```python
from build123d import *

# Parameters (mm, degrees)
SKETCH1_W           = 45
SKETCH1_H           = 45
SKETCH1_R           = 9
SKETCH1_R_2         = 2
BOSS_EXTRUDE1_DEPTH = 15
SKETCH2_R           = 1.65
CUT_EXTRUDE1_DEPTH  = 15
SKETCH3_R           = 3
CUT_EXTRUDE2_DEPTH  = 8
CHAMFER1_SIZE       = 2
SKETCH4_R           = 11.2
CUT_EXTRUDE3_DEPTH  = 2
ECHELLE1_SCALE      = 2
ECHELLE2_SCALE      = 0.25


with BuildPart() as part:
    # Sketch1 → Boss-Extrude1 (new body)
    with BuildSketch(Plane.XY):
        Rectangle(SKETCH1_W, SKETCH1_H)
        Circle(SKETCH1_R, mode=Mode.SUBTRACT)
        with Locations((-17.5, 17.5)):
            Circle(SKETCH1_R_2, mode=Mode.SUBTRACT)
        with Locations((17.5, 17.5)):
            Circle(SKETCH1_R_2, mode=Mode.SUBTRACT)
        with Locations((17.5, -17.5)):
            Circle(SKETCH1_R_2, mode=Mode.SUBTRACT)
        with Locations((-17.5, -17.5)):
            Circle(SKETCH1_R_2, mode=Mode.SUBTRACT)
    extrude(amount=BOSS_EXTRUDE1_DEPTH)

    # Sketch2 → Cut-Extrude1 (cut)
    with BuildSketch(Plane.XY.offset(15)):
        with Locations((9.899494937, 9.899494937)):
            Circle(SKETCH2_R)
        with Locations((9.899494937, -9.899494937)):
            Circle(SKETCH2_R)
        with Locations((-9.899494937, -9.899494937)):
            Circle(SKETCH2_R)
        with Locations((-9.899494937, 9.899494937)):
            Circle(SKETCH2_R)
    extrude(amount=-CUT_EXTRUDE1_DEPTH, mode=Mode.SUBTRACT)

    # Sketch3 → Cut-Extrude2 (cut)
    with BuildSketch(Plane.XY.offset(15)):
        with Locations((9.899494937, 9.899494937)):
            Circle(SKETCH3_R)
        with Locations((9.899494937, -9.899494937)):
            Circle(SKETCH3_R)
        with Locations((-9.899494937, -9.899494937)):
            Circle(SKETCH3_R)
        with Locations((-9.899494937, 9.899494937)):
            Circle(SKETCH3_R)
    extrude(amount=-CUT_EXTRUDE2_DEPTH, mode=Mode.SUBTRACT)

    # Chamfer1
    chamfer1_edges = [part.edges().sort_by_distance(p)[0] for p in [
        (22.5, -22.5, 7.5),
        (-22.5, -22.5, 7.5),
        (-22.5, 22.5, 7.5),
        (22.5, 22.5, 7.5),
    ]]
    chamfer(chamfer1_edges, length=CHAMFER1_SIZE)

    # Sketch4 → Cut-Extrude3 (cut)
    with BuildSketch(Plane(origin=(0, 0, 0), x_dir=(-1, 0, 0), z_dir=(0, 0, -1))):
        Circle(SKETCH4_R)
    extrude(amount=-CUT_EXTRUDE3_DEPTH, mode=Mode.SUBTRACT)


with BuildPart() as part_1:
    # Echelle1: scaled about (0, 0, 7.483766611)
    add(part.part.scale(ECHELLE1_SCALE).moved(Location((0, 0, -7.483766611))))


with BuildPart() as part_2:
    # Echelle2: scaled about (0, 0, 7.483766612)
    add(part_1.part.scale(ECHELLE2_SCALE).moved(Location((0, 0, 5.612824959))))


solid = part_2.part
```
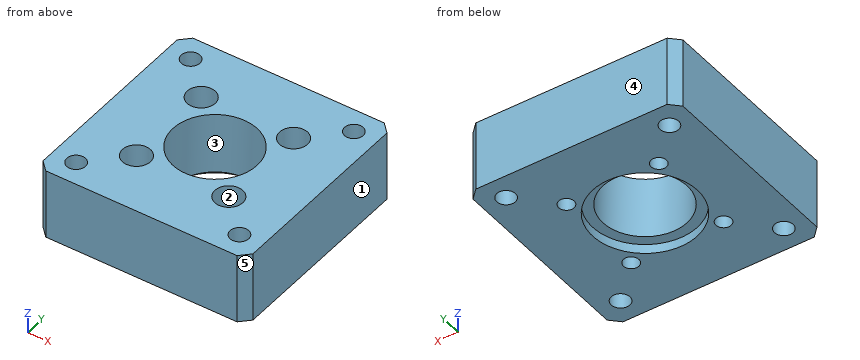
Input: part model. Units: mm. Frame: model coordinates. Face numbers are marked on the shaded views. A direction names the side the tool comes from. Coordinates: 2 decimals unless noted, no trailing zeros. Write each loop counter-clockwise with the first axis right and the second up, starting at its lowest first coordinate (ties: lowest second). Pieces come first, ordered by that corner, then holes.
1) Section C-C on x = 8.75. Output: boundary loops of the cut face in (y, z).
2) Mould query, pull axis Y, two halves, no side actions, for the marked faces 3, 4 and 5. Classes: pulls with the +Y half, pulls with the -Y half, needs draft (parallel to the pull), parting line crosses it, or undercut.
3) Set-up query: the marked faces 1 and 2. Return all of +Z, -Z, +X, -X, +Y, -Y with unobstructed straight access to the full face (end or side cutting, diameter ignored); none if empty.
4) Section A-A on y = 0. Output: boundary loops of the cut face in (x, z).
5) Material intervals for line 1 along X through (y, z) = (0, 9.5); line 2 along Y through (x, z) = (-6.25, 9.5); line 3 along Y through (x, z) = (8.75, 8), sorted ascending.
6) Pin query (flat end, axial travel): pin 1 Ø3.5 at (x, y) = (-4.95, 4.95) entering from -Z; pin 2 Ø0.9 at (x, y) = (-4.5, 5) entering from +Z. Return the tip coordinate at first contact, or that it passes through.
Check result:
1. outline: (-11.25, 3.74) - (-9.75, 3.74) - (-9.75, 11.24) - (-11.25, 11.24) - close; (-7.75, 3.74) - (7.75, 3.74) - (7.75, 11.24) - (-7.75, 11.24) - close; (9.75, 3.74) - (11.25, 3.74) - (11.25, 11.24) - (9.75, 11.24) - close
2. face 3: undercut
2. face 4: pulls with the +Y half
2. face 5: pulls with the -Y half
3. face 1: +Z, -Z, +X, +Y, -Y
3. face 2: +Z
4. outline: (-11.25, 3.74) - (-5.6, 3.74) - (-5.6, 4.74) - (-4.5, 4.74) - (-4.5, 11.24) - (-11.25, 11.24) - close; (4.5, 4.74) - (5.6, 4.74) - (5.6, 3.74) - (11.25, 3.74) - (11.25, 11.24) - (4.5, 11.24) - close
5. line 1: x = -11.25 to -4.5, 4.5 to 11.25
5. line 2: y = -11.25 to -5.7, -4.2 to 4.2, 5.7 to 11.25
5. line 3: y = -11.25 to -9.75, -7.75 to 7.75, 9.75 to 11.25
6. pin 1: stops at z = 3.74
6. pin 2: stops at z = 7.24
